```python
from build123d import *

# Parameters (mm, degrees)
SKETCH1_W           = 26
SKETCH1_H           = 20
SKETCH1_R           = 3.5
SKETCH1_R_2         = 1.6
BOSS_EXTRUDE1_DEPTH = 3
BOSS_EXTRUDE2_START = -9.5
SKETCH2_W           = 5.129495452
SKETCH2_H           = 5
SKETCH2_R           = 1.6
SKETCH2_W_2         = 4.90914111
BOSS_EXTRUDE2_DEPTH = 9.5


with BuildPart() as part:
    # Sketch1 → Boss-Extrude1 (new body)
    with BuildSketch(Plane.XY):
        with Locations((2.16, -1)):
            Rectangle(SKETCH1_W, SKETCH1_H)
        Circle(SKETCH1_R, mode=Mode.SUBTRACT)
        with Locations((-6.34, -8.5)):
            Circle(SKETCH1_R_2, mode=Mode.SUBTRACT)
        with Locations((10.66, -8.5)):
            Circle(SKETCH1_R_2, mode=Mode.SUBTRACT)
    extrude(amount=BOSS_EXTRUDE1_DEPTH)

    # Sketch2 → Boss-Extrude2 (add)
    # profile 1 of 2: a face of its own
    with BuildSketch(Plane.XY.offset(BOSS_EXTRUDE2_START)):
        with Locations((-6.34, -8.5)):
            Rectangle(SKETCH2_W, SKETCH2_H)
        with Locations((-6.34, -8.5)):
            Circle(SKETCH2_R, mode=Mode.SUBTRACT)
    # profile 2 of 2: a face of its own
    with BuildSketch(Plane.XY.offset(BOSS_EXTRUDE2_START)):
        with Locations((10.66, -8.5)):
            Rectangle(SKETCH2_W_2, SKETCH2_H)
        with Locations((10.66, -8.5)):
            Circle(SKETCH2_R, mode=Mode.SUBTRACT)
    extrude(amount=BOSS_EXTRUDE2_DEPTH)


solid = part.part
```
For this review, take the finished solid that the model builds, in its own axes (mm). A direction names the side the tool comes from. Coordinates: 2 decimals unless noted, no trailing zeros. Loops run counter-clockwise (first coordinate to the right, second up) from the corner with the lowest first, then second, coordinate; pieces in that order, holes last. Notation, with made-up numbers: (83, 29.5) -> (141, 29.5) arc R5 cw to (141, 36.5) -> close; hole circle Ø4 at (31.5, 83). An arc over 180 degrees is marked (long way). Return JSON: item names as keys, results as strings. Group by question number.
(1) To check wall thickness, follow L1, parallel to Y at x = -6.34, z = -2; L2, parallel to Y at x = 0, z = 1.4; L3, parallel to X at y = -9.5, z = -1. State the ranges of each line that lie inside material, in increasing order.
(2) Tool access review of faces 1 (the flat face through (13.115, -9, -5)), 2 (the flat face through (11, -6, -5)), 3 (the cylindrical face through (9.06, -8.43, -3.34)), 4 (the flat face through (-3.775, -9, -5)), 5 (the flat face through (-8.905, -9, -5)): name each direction out of +Z, -Z, +X, -X, +Y, -Y from which nothing blocks a thin tool from reaching the whole face with its end or side.
(3) Consider section C-C, the plane x = -6.34. Give the boundary of the cut face in (y, z), plus the area to 3 significant figures.
(4) Consider section A-A, the plane y = 0. Give the boundary of the cut face in (x, z).
(5) Consider section D-D, the plane z = 1.75. Give the boundary of the cut face in (x, y).
(6) For pin 1 Ø8 at (x, y) = (10.5, 2) entering from -Z; pin 2 Ø1.5 at (x, z) = (11.5, -2.5) entering from +Y; pin 3 Ø2.5 at (y, z) = (-8, -4.5) entering from -X, all flat-tipped, find the tip position at first contact; note any pin that passes through.
(7) Mouldability with a two-part tool opening along Y and no side actions: class faces 6 (the flat face through (2, 9, 1)), 7 (the cylindrical face through (-6.69, -10.06, -3.34)), 8 (the flat face through (-10.84, -1, 1)) as pulls with the +Y half, pulls with the -Y half, needs draft (parallel to the pull), parting line crosses it, or undercut.
(8) Consider section B-B, the plane z = -7.5. Give the boundary of the cut face in (x, y), plus the area to 3 significant figures.
Results below:
{
 "1": {"L1": "y = -11 to -10.1, -6.9 to -6", "L2": "y = -11 to -3.5, 3.5 to 9", "L3": "x = -8.9 to -7.59, -5.09 to -3.78, 8.21 to 9.41, 11.91 to 13.11"},
 "2": {"face 1": "-Z, +X, +Y, -Y", "face 2": "-Z, +X, -X, +Y", "face 3": "+Z, -Z", "face 4": "-Z, +Y, -Y", "face 5": "-Z, -X, +Y, -Y"},
 "3": {"outline": "(-11, -9.5) -> (-10.1, -9.5) -> (-10.1, 3) -> (-11, 3) -> close; (-6.9, -9.5) -> (-6, -9.5) -> (-6, 0) -> (9, 0) -> (9, 3) -> (-6.9, 3) -> close", "area": "67.5 mm2"},
 "4": {"outline": "(-10.84, 0) -> (-3.5, 0) -> (-3.5, 3) -> (-10.84, 3) -> close; (3.5, 0) -> (15.16, 0) -> (15.16, 3) -> (3.5, 3) -> close"},
 "5": {"outline": "(-10.84, -11) -> (15.16, -11) -> (15.16, 9) -> (-10.84, 9) -> close; hole circle Ø3.2 at (-6.34, -8.5); hole circle Ø7 at (0, 0); hole circle Ø3.2 at (10.66, -8.5)"},
 "6": {"pin 1": "stops at z = 0", "pin 2": "stops at y = -6", "pin 3": "stops at x = -8.9"},
 "7": {"face 6": "pulls with the +Y half", "face 7": "undercut", "face 8": "needs draft"},
 "8": {"outline": "(-8.9, -11) -> (-3.78, -11) -> (-3.78, -6) -> (-8.9, -6) -> close; (8.21, -11) -> (13.11, -11) -> (13.11, -6) -> (8.21, -6) -> close; hole circle Ø3.2 at (-6.34, -8.5); hole circle Ø3.2 at (10.66, -8.5)", "area": "34.1 mm2"}
}
